Here's how the part is built. I have some questions about the finished solid (model axes, mm). Round coordinates to 2 decimals unless told otherwise and drop trailing zeros. Write each loop counter-clockwise with the first axis right and the second up, starting at its lowest first coordinate (ties: lowest second). Pieces come first, ordered by that corner, then holes. Notation, with made-up numbers: (-20.5, 83) -> (-16.5, 83) arc R5 cw to (-16.5, 92) -> close; hole circle Ø5 at (19.25, 74). An arc over 180 degrees is marked (long way). Put each result on its own line as item: value. Start each with the question number.
1) I want a section at B-B, the plane y = 6.5. List the corners of the cut face in (x, z) for me, then the cut area to 3 significant figures.
2) Will these pins go through, and if not, where does the flat tip stop? P1, Ø1, axis at y = 6, z = 53, coming from the +X side; P2, Ø10.5, axis at x = -71, z = 87.5, coming from the +Y side; P3, Ø2.5, axis at y = 7, z = -2, coming from the -X side; P4, Ø3, axis at x = -7.5, y = 7, coming from the +Z side.
3) If I drill on line 1 along X through (y, z) = (3.9, -87.5); line 2 along Y through (x, z) = (217.5, 74); line 3 along Z through (x, y) = (69.5, 1.5), over which ranges is the centre line in solid material (lowest first)? Write a range as [from, to].
4) I want a section at A-A, the plane x = 147.5. List the corners of the cut face in (y, z) for me.
from build123d import *

# Parameters (mm, degrees)
SKETCH2_R           = 4
SKETCH2_W           = 30
SKETCH2_H           = 10
BOSS_EXTRUDE1_DEPTH = 5
SKETCH2_2_W         = 30
SKETCH2_2_H         = 10
BOSS_EXTRUDE2_DEPTH = 10


with BuildPart() as part:
    # Sketch2 → Boss-Extrude1 (new body)
    with BuildSketch(Plane(origin=(0, 0, 0), x_dir=(1, 0, 0), z_dir=(0, 1, 0))):
        with BuildLine():
            Line((-227.9, -94.4), (227.9, -94.4))
            ThreePointArc((227.9, -94.4), (244.163455967, -87.663455967), (250.9, -71.4))
            Line((250.9, -71.4), (250.9, 71.4))
            ThreePointArc((250.9, 71.4), (244.163455967, 87.663455967), (227.9, 94.4))
            Line((227.9, 94.4), (-227.9, 94.4))
            ThreePointArc((-227.9, 94.4), (-244.163455967, 87.663455967), (-250.9, 71.4))
            Line((-250.9, 71.4), (-250.9, -71.4))
            ThreePointArc((-250.9, -71.4), (-244.163455967, -87.663455967), (-227.9, -94.4))
        make_face()
        with Locations(Location((-213, 87.5, 0), (0, 0, 270))):
            Circle(SKETCH2_R, mode=Mode.SUBTRACT)
        with Locations(Location((-71, 87.5, 0), (0, 0, 270))):
            Circle(SKETCH2_R, mode=Mode.SUBTRACT)
        with Locations(Location((71, 87.5, 0), (0, 0, 270))):
            Circle(SKETCH2_R, mode=Mode.SUBTRACT)
        with Locations(Location((213, 87.5, 0), (0, 0, 270))):
            Circle(SKETCH2_R, mode=Mode.SUBTRACT)
        with Locations(Location((213, -87.5, 0), (0, 0, 90))):
            Circle(SKETCH2_R, mode=Mode.SUBTRACT)
        with Locations(Location((71, -87.5, 0), (0, 0, 90))):
            Circle(SKETCH2_R, mode=Mode.SUBTRACT)
        with Locations(Location((-71, -87.5, 0), (0, 0, 90))):
            Circle(SKETCH2_R, mode=Mode.SUBTRACT)
        with Locations(Location((-213, -87.5, 0), (0, 0, 90))):
            Circle(SKETCH2_R, mode=Mode.SUBTRACT)
        Rectangle(SKETCH2_W, SKETCH2_H, mode=Mode.SUBTRACT)
    extrude(amount=BOSS_EXTRUDE1_DEPTH)

    # Sketch2_2 → Boss-Extrude2 (add)
    with BuildSketch(Plane(origin=(0, 0, 0), x_dir=(1, 0, 0), z_dir=(0, 1, 0))):
        Rectangle(SKETCH2_2_W, SKETCH2_2_H)
    extrude(amount=BOSS_EXTRUDE2_DEPTH)


solid = part.part
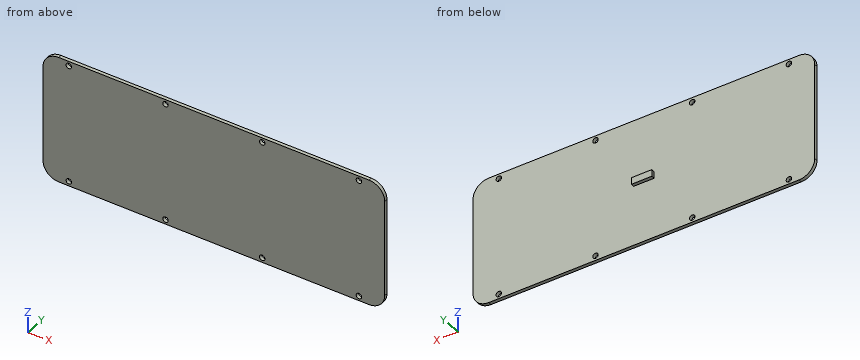
Findings:
1. outline: (-15, -5) -> (15, -5) -> (15, 5) -> (-15, 5) -> close
1. area: 300 mm2
2. P1: passes through
2. P2: stops at y = 5
2. P3: stops at x = -15
2. P4: stops at z = 5
3. line 1: x = [-244.33, -217], [-209, -75], [-67, 67], [75, 209], [217, 244.33]
3. line 2: y = [0, 5]
3. line 3: z = [-94.4, -91.21], [-83.79, 83.79], [91.21, 94.4]
4. outline: (0, -94.4) -> (5, -94.4) -> (5, 94.4) -> (0, 94.4) -> close
